from build123d import *

# Parameters (mm, degrees)
BOSS_EXTRUDE1_DEPTH = 7.62
SKETCH2_R           = 6.35
CUT_EXTRUDE1_DEPTH  = 18.289422585
CHAMFER1_SIZE       = 0.9906


with BuildPart() as part:
    # Sketch1 → Boss-Extrude1 (new body)
    with BuildSketch(Plane(origin=(0, 0, 0), x_dir=(1, 0, 0), z_dir=(0, 1, 0))):
        Polygon((0, -11.73175747), (10.16, -5.865878735), (10.16, 5.865878735), (0, 11.73175747), (-10.16, 5.865878735), (-10.16, -5.865878735), align=None)
    extrude(amount=BOSS_EXTRUDE1_DEPTH)

    # Sketch2 → Cut-Extrude1 (cut, through all)
    with BuildSketch(Plane(origin=(0, 7.62, 0), x_dir=(1, 0, 0), z_dir=(0, 1, 0))):
        with Locations(Location((0, 0, 0), (0, 0, 270))):
            Circle(SKETCH2_R)
    extrude(amount=-CUT_EXTRUDE1_DEPTH, mode=Mode.SUBTRACT)

    # Chamfer1
    chamfer1_edges = [part.edges().sort_by_distance(p)[0] for p in [
        (0, 0, -6.35),
        (0, 7.62, -6.35),
    ]]
    chamfer(chamfer1_edges, length=CHAMFER1_SIZE)

    # Sketch3 → Cut-Revolve1 (revolve, cut)
    with BuildSketch(Plane(origin=(0, 0, 0), x_dir=(0, 0, -1), z_dir=(1, 0, 0))):
        Polygon((-11.73175747, 7.62), (-10.46175747, 7.62), (-11.73175747, 6.604), align=None)
        Polygon((-11.73175747, 0), (-11.73175747, 1.016), (-10.46175747, 0), align=None)
    revolve(axis=Axis((0, 10.605597555, 0), (0, -1, 0)), mode=Mode.SUBTRACT)


solid = part.part
Input: part model. Units: mm. Frame: model coordinates. Round coordinates to 2 decimals unless told otherwise and drop trailing zeros. Write each loop counter-clockwise with the first axis right and the second up, starting at its lowest first coordinate (ties: lowest second). Pieces come first, ordered by that corner, then holes.
1) Ray query, L1, parallel to X at y = 5, z = 0; L2, parallel to Z at x = 5.5, y = 4.75; L3, parallel to Z at x = -4.25, y = 1.5. Return the intervals inside material, ascending.
2) Cut plane C-C (y = 0.5). Return the cut outline in (x, z).
3) Contact query for a flat-ended pin moving along its axis: P1, Ø1.5, axis at y = 5.5, z = 6, coming from the -X side. Output: stop coordinate, or through.
4) Cut plane B-B (z = 0). Return the cut outline in (x, y).
5) Cut plane A-A (y = 3). Return the cut outline in (x, z), then the cut area to 3 significant figures.
6) Draft query along Z for faces 1 (the cylindrical face through (-3.86, 3.85, -5.04)), 2 (the flat face through (-2.4, 7.62, -7.1)), 3 (the flat face through (5.01, 3.76, 8.84)). Return one class per face: pulls with the +Z half, pulls with the -Z half, needs draft (parallel to the pull), parting line crosses it, or undercut.
Geometry says:
1. L1: x = -10.16 to -6.35, 6.35 to 10.16
1. L2: z = -8.56 to -3.17, 3.17 to 8.56
1. L3: z = -9.28 to -4.72, 4.72 to 9.28
2. outline: (-10.16, -4.44) arc R11.09 ccw to (-8.92, -6.58) - (-1.24, -11.02) arc R11.09 ccw to (1.24, -11.02) - (8.92, -6.58) arc R11.09 ccw to (10.16, -4.44) - (10.16, 4.44) arc R11.09 ccw to (8.92, 6.58) - (1.24, 11.02) arc R11.09 ccw to (-1.24, 11.02) - (-8.92, 6.58) arc R11.09 ccw to (-10.16, 4.44) - close; hole circle Ø13.68 at (0, 0)
3. P1: stops at x = -10.16
4. outline: (-10.16, 0) - (-7.34, 0) - (-6.35, 0.99) - (-6.35, 6.63) - (-7.34, 7.62) - (-10.16, 7.62) - close; (6.35, 0.99) - (7.34, 0) - (10.16, 0) - (10.16, 7.62) - (7.34, 7.62) - (6.35, 6.63) - close
5. outline: (-10.16, -5.87) - (0, -11.73) - (10.16, -5.87) - (10.16, 5.87) - (0, 11.73) - (-10.16, 5.87) - close; hole circle Ø12.7 at (0, 0)
5. area: 231 mm2
6. face 1: undercut
6. face 2: needs draft
6. face 3: pulls with the +Z half
